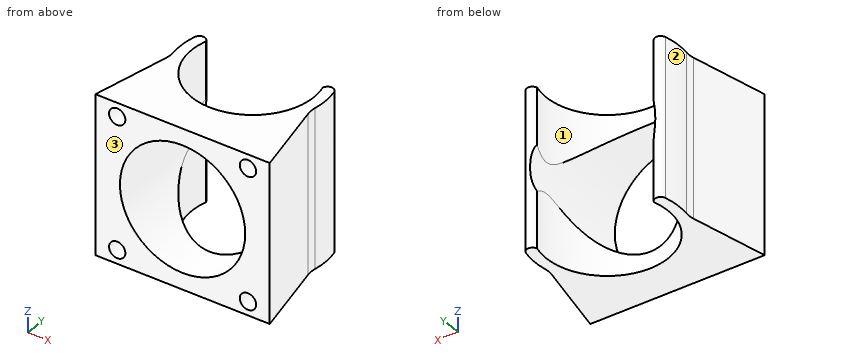
from build123d import *

# Parameters (mm, degrees)
F1_DEPTH = 29
F2_R     = 11.5
F3_DEPTH = 25
F2_R_2   = 1.5
F4_DEPTH = 8


# Not quite as in the source:
# - a feature names something its author has since deleted; it is built from what else it names


with BuildPart() as f1:
    # F0 (on Top) → F1 (new body)
    with BuildSketch(Plane.XY):
        with BuildLine():
            ThreePointArc((10.7388314076, 3), (0, -11.15), (-10.7388314076, 3))
            ThreePointArc((-10.7388314076, 3), (-11.7710268291, 3.8182927175), (-12.8032222507, 3))
            ThreePointArc((-12.8032222507, 3), (-13.142833705, 0.4340762628), (-12.9732702789, -2.148664299))
            ThreePointArc((-12.9732702789, -2.148664299), (-12.9072730339, -3.0752015435), (-13.0137997447, -3.9979577203))
            Line((-13.0137997447, -3.9979577203), (-16, -18.15))
            Line((-16, -18.15), (0, -18.15))
            Line((0, -18.15), (16, -18.15))
            Line((16, -18.15), (13.0137997447, -3.9979577203))
            ThreePointArc((13.0137997447, -3.9979577203), (12.9072730339, -3.0752015435), (12.9732702789, -2.148664299))
            ThreePointArc((12.9732702789, -2.148664299), (13.142833705, 0.4340762628), (12.8032222507, 3))
            ThreePointArc((12.8032222507, 3), (11.7710268291, 3.8182927175), (10.7388314076, 3))
        make_face()
    extrude(amount=F1_DEPTH)

    # F2 (on face) → F3 (cut)
    with BuildSketch(Plane.XZ.offset(18.15)):
        with Locations((0, 14.5)):
            Circle(F2_R)
    extrude(amount=-F3_DEPTH, mode=Mode.SUBTRACT)

    # F2 (on face) → F4 (cut)
    with BuildSketch(Plane.XZ.offset(18.15)):
        with Locations((-12, 26.5)):
            Circle(F2_R_2)
        with Locations((-12, 2.5)):
            Circle(F2_R_2)
        with Locations((12, 26.5)):
            Circle(F2_R_2)
        with Locations((12, 2.5)):
            Circle(F2_R_2)
    extrude(amount=-F4_DEPTH, mode=Mode.SUBTRACT)


solid = f1.part
Build history of the part. All positions in model axes, mm. Face numbers are marked on the shaded views. Coordinates: 2 decimals unless noted, no trailing zeros. Write each loop counter-clockwise with the first axis right and the second up, starting at its lowest first coordinate (ties: lowest second). Pieces come first, ordered by that corner, then holes.
(1) Mould opens along X. For the marked faces 1, 2 and 3 say: pulls with the +X half, pulls with the -X half, needs draft (parallel to the pull), parting line crosses it, or undercut.
(2) Pin check, flat tips, straight feed: pin 1 Ø3 at (y, z) = (0, 19.5) entering from -X; pin 2 Ø6 at (y, z) = (-9.5, 22.5) entering from -X; pin 3 Ø8 at (x, z) = (-1.5, 19) entering from +Y (3 decimals); pin 4 Ø0.9 at (x, z) = (12, 26) entering from -Y. Stop position of each tip, or through.
(3) Cut at B-B on x = 6. List the corners of the cut face in (y, z).
(4) Cut at D-D on y = -16.5. List the corners of the cut face in (x, z), and give its area (3 significant figures).
(5) Drill centre lines: line 1 (Z direction, x = -12, y = -15); line 2 (X direction, y = -10.25, z = 19.25); line 3 (Y direction, x = 11.5, z = 22.5). Where is each one in solid material? Low to high.
(6) Cut at C-C on z = 6. List the corners of the cut face in (x, y), and give its area (3 significant figures).
(7) Cut at A-A on y = 0. List the corners of the cut face in (x, z), and give its area (3 significant figures).
Working result:
1. face 1: undercut
1. face 2: pulls with the -X half
1. face 3: needs draft
2. pin 1: stops at x = -13.15
2. pin 2: stops at x = -14.81
2. pin 3: passes through
2. pin 4: stops at y = -10.15
3. outline: (-18.15, 0) - (-9.4, 0) - (-9.4, 4.69) - (-18.15, 4.69) - close; (-18.15, 24.31) - (-9.4, 24.31) - (-9.4, 29) - (-18.15, 29) - close
4. outline: (-15.65, 0) - (15.65, 0) - (15.65, 29) - (-15.65, 29) - close; hole circle Ø3 at (-12, 2.5); hole circle Ø3 at (-12, 26.5); hole circle Ø23 at (0, 14.5); hole circle Ø3 at (12, 2.5); hole circle Ø3 at (12, 26.5)
4. area: 464 mm2
5. line 1: z = 0 to 1, 4 to 25, 28 to 29
5. line 2: x = -14.33 to -10.47, 10.47 to 14.33
5. line 3: y = -18.15 to 3.78
6. outline: (-16, -18.15) - (-7.75, -18.15) - (-7.75, -8.02) arc R11.15 cw to (-10.74, 3) arc R1.06 ccw to (-12.8, 3) arc R13.15 ccw to (-12.97, -2.15) arc R5 cw to (-13.01, -4) - close; (7.75, -18.15) - (16, -18.15) - (13.01, -4) arc R5 cw to (12.97, -2.15) arc R13.15 ccw to (12.8, 3) arc R1.06 ccw to (10.74, 3) arc R11.15 cw to (7.75, -8.02) - close
6. area: 210 mm2
7. outline: (-13.15, 0) - (-11.15, 0) - (-11.15, 11.68) arc R11.5 cw to (-11.15, 17.32) - (-11.15, 29) - (-13.15, 29) - close; (11.15, 0) - (13.15, 0) - (13.15, 29) - (11.15, 29) - (11.15, 17.32) arc R11.5 cw to (11.15, 11.68) - close
7. area: 113 mm2
